Could you check a few things on this model? Use its own coordinates, in mm. A direction names the side the tool comes from. Round coordinates to 2 decimals unless told otherwise and drop trailing zeros. Loops run counter-clockwise (first coordinate to the right, second up) from the corner with the lowest first, then second, coordinate; pieces in that order, holes last. Notation, with made-up numbers: (79.5, -40) - (113.5, -40) arc R26 cw to (113.5, -13) - close; hole circle Ø8 at (-34, 47). An arc over 180 degrees is marked (long way). Use one line per item in the form item = value.
```python
from build123d import *

# Parameters (mm, degrees)
F0_R     = 2.25
F1_DEPTH = 1


with BuildPart() as f1:
    # F0 (on Top) → F1 (new body)
    with BuildSketch(Plane.XY):
        with BuildLine():
            Line((21.677962, 62.992528), (10.139461, 66.734109))
            Line((10.139461, 66.734109), (-10.943207, 62.093519))
            Line((-10.943207, 62.093519), (-21.901843, 20.660526))
            ThreePointArc((-21.901843, 20.660526), (-24.475691, 15.352547), (-28.134067, 10.724846))
            Line((-28.134067, 10.724846), (-57.256493, -18.85125))
            Line((-57.256493, -18.85125), (-65.39211, -12.722599))
            Line((-65.39211, -12.722599), (-62.863164, -24.586024))
            Line((-62.863164, -24.586024), (-48.302961, -40.523855))
            Line((-48.302961, -40.523855), (-6.941619, -29.297815))
            ThreePointArc((-6.941619, -29.297815), (-1.048655, -28.621876), (4.779045, -29.72724))
            Line((4.779045, -29.72724), (44.953908, -40.159952))
            Line((44.953908, -40.159952), (43.714149, -50.269929))
            Line((43.714149, -50.269929), (52.723703, -42.148085))
            Line((52.723703, -42.148085), (59.246168, -21.569664))
            Line((59.246168, -21.569664), (28.843462, 8.637289))
            ThreePointArc((28.843462, 8.637289), (25.3116, 13.402776), (23.355023, 19.002394))
            Line((23.355023, 19.002394), (12.302585, 59.011202))
            Line((12.302585, 59.011202), (21.677962, 62.992528))
        make_face()
        Polygon((-47.492523, -37.312847), (-60.201257, -23.785029), (-56.482609, -22.158133), (-49.804259, -15.479784), (-38.642525, -34.910835), align=None, mode=Mode.SUBTRACT)
        Polygon((-22.399317, -12.932252), (-23.90843, -27.290503), (-38.03028, -30.292195), (-45.24895, -17.789091), (-35.588484, -7.060056), align=None, mode=Mode.SUBTRACT)
        Polygon((-21.780303, 8.790208), (-13.818382, 11.310016), (-7.655204, 5.674693), (-9.453948, -2.480436), (-17.415869, -5.000244), (-23.579047, 0.635079), align=None, mode=Mode.SUBTRACT)
        Polygon((47.430811, -37.836308), (38.308016, -35.391861), (49.554932, -16.009991), (56.060134, -22.473308), (50.699068, -40.243304), align=None, mode=Mode.SUBTRACT)
        Polygon((3.277608, -23.2574), (-2.88557, -17.622078), (-1.086826, -9.466948), (6.875095, -6.947141), (13.038273, -12.582463), (11.239529, -20.737593), align=None, mode=Mode.SUBTRACT)
        Circle(F0_R, mode=Mode.SUBTRACT)
        Polygon((22.399317, -12.932252), (35.588484, -7.060056), (45.24895, -17.789091), (38.03028, -30.292195), (23.90843, -27.290503), align=None, mode=Mode.SUBTRACT)
        Polygon((18.502695, 14.467192), (16.703952, 6.312062), (8.742031, 3.792255), (2.578853, 9.427577), (4.377597, 17.582707), (12.339518, 20.102514), align=None, mode=Mode.SUBTRACT)
        Polygon((-11.680054, 34.350559), (-7.21867, 48.081286), (7.21867, 48.081286), (11.680054, 34.350559), (0, 25.864504), align=None, mode=Mode.SUBTRACT)
        Polygon((9.051799, 59.994441), (11.496243, 50.871646), (-10.912408, 50.920826), (-8.567612, 59.786155), (9.50219, 64.028333), align=None, mode=Mode.SUBTRACT)
    extrude(amount=F1_DEPTH)


solid = f1.part
```
1. If we section it at A-A, the plane y = 53: Write out the boundary of the cut face in (x, z).
Solution:
outline = (-13.35, 0) - (-10.36, 0) - (-10.36, 1) - (-13.35, 1) - close; (10.93, 0) - (13.96, 0) - (13.96, 1) - (10.93, 1) - close
2. We'd pull the mould along X, two halves only. Please class faces 4 (the face through (43.85, -25.84, 0.49)), 5 (the face through (48.156, -46.266, 0.493)), 6 (the face through (-16.346, 41.667, 0.493)): +X half, -X half, draft (parallel to the pull), parting line (faces both ways), or undercut.
Solution:
face_4 = undercut
face_5 = +X half
face_6 = -X half
3. Please list where these lines run through material, in increasing order: line 1 along Y through (x, z) = (0, 0.7); line 2 along Y through (x, z) = (39, 0.65); line 3 along Y through (x, z) = (43.5, 0.3).
Solution:
line_1 = -28.69 to -20.26, -9.12 to -2.25, 2.25 to 25.86, 48.08 to 50.9, 61.8 to 64.5
line_2 = -38.61 to -35.58, -34.2 to -28.61, -10.85 to -1.45
line_3 = -39.78 to -36.78, -26.44 to -20.82, -15.85 to -5.92
4. On a 3-axis mill with a long thin cutter (end or side, diameter ignored), from which of +Z, -Z, +X, -X, +Y, -Y can I reach the whole of each face in a straight line? I mean faces 1 (the face through (0.24, -20.48, 0.49)), 2 (the face through (44.26, -6.68, 0.49)), 3 (the face through (-42.491, -3.856, 0.493)). Say none if no direction works.
Solution:
face_1 = +Z, -Z
face_2 = +Z, -Z, +X, +Y
face_3 = +Z, -Z, +Y
5. If we section it at B-B, the plane z = 0.3: Count the separate pieces of the cut face and the enclosed holes in it, plus the area to 3 significant figures.
Solution:
separate_pieces = 1
enclosed_holes = 10
area = 4,130 mm^2
6. If we section it at C-C, the plane y = 23: Write out the boundary of the cut face in (x, z), plus the area to 3 significant figures.
Solution:
outline = (-21.28, 0) - (22.25, 0) - (22.25, 1) - (-21.28, 1) - close
area = 43.5 mm^2
